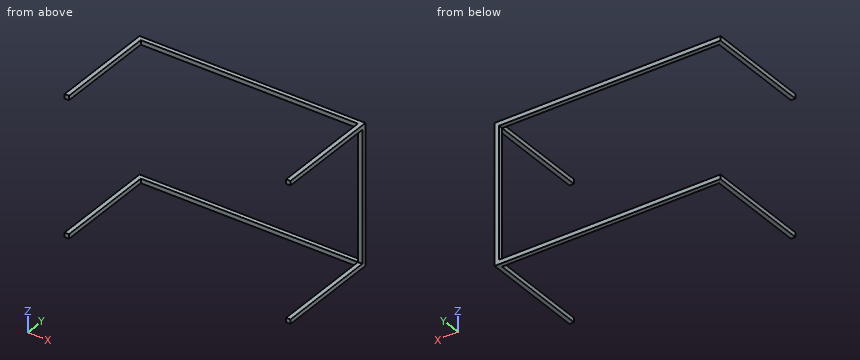
```python
from build123d import *

# Parameters (mm, degrees)
SKETCH1_W           = 1270
SKETCH1_H           = 25.4
BOSS_EXTRUDE1_DEPTH = 25.4
SKETCH2_W           = 25.4
SKETCH2_H           = 25.4
BOSS_EXTRUDE2_DEPTH = 584.2


with BuildPart() as part:
    # Sketch1 → Boss-Extrude1 (new body)
    with BuildSketch(Plane(origin=(0, 0, 0), x_dir=(1, 0, 0), z_dir=(0, 1, 0))):
        with Locations((114.3, -387.35)):
            Rectangle(SKETCH1_W, SKETCH1_H)
        Polygon((749.3, 374.65), (749.3, -374.65), (749.3, -400.05), (774.7, -400.05), (774.7, 400.05), (749.3, 400.05), align=None)
        with Locations((114.3, 387.35)):
            Rectangle(SKETCH1_W, SKETCH1_H)
    extrude(amount=BOSS_EXTRUDE1_DEPTH)

    # Sketch2 → Boss-Extrude2 (add)
    with BuildSketch(Plane(origin=(0, 0, 0), x_dir=(1, 0, 0), z_dir=(0, 1, 0))):
        with Locations((-508, 387.35)):
            Rectangle(SKETCH2_W, SKETCH2_H)
        with Locations((762, 387.35)):
            Rectangle(SKETCH2_W, SKETCH2_H)
        with Locations((762, -387.35)):
            Rectangle(SKETCH2_W, SKETCH2_H)
        with Locations((-508, -387.35)):
            Rectangle(SKETCH2_W, SKETCH2_H)
    extrude(amount=-BOSS_EXTRUDE2_DEPTH)


solid = part.part
```
CAD build for the part. Positions are in the model's coordinates, mm. Coordinates: 2 decimals unless noted, no trailing zeros. Order: outer loops, then holes, each group sorted by start corner. A loop starts at its lowest first (then second) coordinate and runs counter-clockwise, first axis right, second up. Notation, with made-up numbers: (51, 31) - (78, 31) arc R10 ccw to (78, 44) - close; hole circle Ø5 at (30, -35). An arc over 180 degrees is marked (long way). Use a Markdown table: item, result. Add a question column.
(1) Flat gauge pins, fed straight in: pin 1 (20.5 mm diameter, centred on x = 756, z = 82.5, fed in from -Y); pin 2 (12.5 mm diameter, centred on y = 12.5, z = 186, fed in from -X). Where does each tip first touch, or does it go through?
(2) Saw through at B-B (x = 287.5). Give the cut face in (y, z).
(3) Saw through at C-C (z = 351). Give the cut face in (x, y).
(4) Saw through at A-A (y = -263.5). Give the cut face in (x, z), then the cut area to 3 significant figures.
Solved:
| question | item | result |
|---|---|---|
| 1 | pin 1 | stops at y = 0 |
| 1 | pin 2 | stops at x = 749.3 |
| 2 | outline | (0, -400.05) - (25.4, -400.05) - (25.4, -374.65) - (0, -374.65) - close; (0, 374.65) - (25.4, 374.65) - (25.4, 400.05) - (0, 400.05) - close |
| 3 | outline | (749.3, 0) - (774.7, 0) - (774.7, 25.4) - (749.3, 25.4) - close |
| 4 | outline | (-520.7, -400.05) - (-495.3, -400.05) - (-495.3, -374.65) - (-520.7, -374.65) - close; (-520.7, 374.65) - (-495.3, 374.65) - (-495.3, 400.05) - (-520.7, 400.05) - close; (749.3, -400.05) - (774.7, -400.05) - (774.7, -374.65) - (749.3, -374.65) - close; (749.3, 374.65) - (774.7, 374.65) - (774.7, 400.05) - (749.3, 400.05) - close |
| 4 | area | 2,580 mm² |
